```python
from build123d import *

# Parameters (mm, degrees)
F0_W     = 480
F0_H     = 185
F1_DEPTH = 265
F3_DEPTH = 480
F5_W     = 472
F5_H     = 257
F6_DEPTH = 181


with BuildPart() as f1:
    # F0 (on Front) → F1 (new body)
    with BuildSketch(Plane.XZ):
        with Locations((-240, 92.5)):
            Rectangle(F0_W, F0_H)
    extrude(amount=-F1_DEPTH)

    # F2 (on Right) → F3 (cut, through all)
    with BuildSketch(Plane.YZ):
        Polygon((0, 50), (4, 50), (261, 185), (0, 185), align=None)
    extrude(amount=-F3_DEPTH, mode=Mode.SUBTRACT)

    # F5 (on plane+point) → F6 (cut)
    with BuildSketch(Plane.XY.offset(185)):
        with Locations((-240, 132.5)):
            Rectangle(F5_W, F5_H)
    extrude(amount=-F6_DEPTH, mode=Mode.SUBTRACT)


solid = f1.part
```
Verification items for the finished model (mm, model axes). A direction names the side the tool comes from. Give positions to 0.01 mm unless a question says otherwise; leave off trailing zeros. Write each loop counter-clockwise with the first axis right and the second up, starting at its lowest first coordinate (ties: lowest second). Pieces come first, ordered by that corner, then holes. Notation, with made-up numbers: M 40,82.25 L 69,82.25 A16 cw 69,100.25 Z; hole C 43,69.5 d10. An arc over 180 degrees is marked long. One line per question, with ' | ' between items.
1) Set-up check for faces 1 (the flat face through (-243, 134, 4)), 2 (the flat face through (-243, 131, 0)): record each of +Z, -Z, +X, -X, +Y, -Y from which the full face is reachable in a straight line by a thin tool's end or side.
Result:
face 1: +Z | face 2: -Z, +X, -X, +Y, -Y
2) Mould release check, pull along X, two halves, no side actions. Record for faces 3 (the flat face through (-4, 159, 76)), 4 (the flat face through (-1.972, 130.701, 116.555)), 5 (the flat face through (0, 160, 71)): released by +X, released by -X, zero draft, split by the parting line, or undercut.
Result:
face 3: undercut | face 4: zero draft | face 5: released by +X
3) Section check C-C on y = 44. Enter the section's corners in (x, z).
Result:
outline: M -480,0 L 0,0 L 0,71.01 L -4,71.01 L -4,4 L -476,4 L -476,71.01 L -480,71.01 Z
4) Section check A-A on z = 24. Enter the section's corners in (x, y), plus the area to 3 significant figures.
Result:
outline: M -480,0 L 0,0 L 0,265 L -480,265 Z; hole M -476,4 L -4,4 L -4,261 L -476,261 Z | area: 5,900 mm2
5) Thickness scan on line 1 along X through (y, z) = (173, 75); line 2 along Y through (x, z) = (-253.5, 42); line 3 along Z through (x, y) = (-227, 73). Record the ranges inside material, lowest first. Write a range as [from, to].
Result:
line 1: x = [-480, -476], [-4, 0] | line 2: y = [0, 4], [261, 265] | line 3: z = [0, 4]
6) Section check B-B on x = -147. Enter the section's corners in (y, z), plus the area to 3 significant figures.
Result:
outline: M 0,0 L 265,0 L 265,185 L 261,185 L 261,4 L 4,4 L 4,50 L 0,50 Z | area: 1,970 mm2
7) Gauge pin test, flat ends, axial feed: pin 1 Ø10 at (x, z) = (-380.5, 135) entering from -Y; pin 2 Ø6 at (x, z) = (-61, 37.5) entering from -Y; pin 3 Ø2 at (x, y) = (-221.5, 48) entering from +Z; pin 4 Ø1.2 at (x, y) = (-144, 3) entering from +Z. Record the tip position at first contact, or that the pin passes through.
Result:
pin 1: stops at y = 261 | pin 2: stops at y = 0 | pin 3: stops at z = 4 | pin 4: stops at z = 50
